For this review, use the dimensioned drawing (mm, ordinates from the lowest corner) and the shaded views. A direction names the side the tool comes from. Give positions to 0.01 mm unless a question says otherwise; leave off trailing zeros. Write each loop counter-clockwise with the first axis right and the second up, starting at its lowest first coordinate (ties: lowest second). Pieces come first, ordered by that corner, then holes. Notation, with made-up numbers: M -23.75,65.25 L 2.25,65.25 A22 ccw 2.25,103.25 Z; hole C 24.25,51.25 d6. An arc over 180 degrees is marked long. One line per item, written item: value. Start each with the question number.
Item 1: Consider section A-A, the plane x = 27.5. Write out the cut boundary in (y, z), and give its area (3 significant figures).
Item 2: Consider section B-B, the plane y = 15. Write out the cut boundary in (x, z), and give its area (3 significant figures).
Item 3: Tool access review of the marked faces 1 and 2: name each direction out of +Z, -Z, +X, -X, +Y, -Y from which nothing blocks a thin tool from reaching the whole face with its end or side.
Item 4: Mouldability with a two-part tool opening along X and no side actions: class the marked faces 3, 4 and 5 as released by +X, released by -X, zero draft, split by the parting line, or undercut.
Item 5: Clearance check with flat-ended pins moving along their axes: pin 1 Ø6 at (y, z) = (8.5, 13) entering from -X; pin 2 Ø11 at (x, y) = (15.5, 12.5) entering from -Z; pin 3 Ø6 at (x, y) = (5.5, 8.5) entering from +Z. State where each tip first meets the part, or that it passes through.
Item 6: Consider section D-D, the plane x = 15. Write out the cut boundary in (y, z), and give its area (3 significant figures).
Item 7: To check wall thickness, follow probe 1 along Y at (x, z) = (15, 7); probe 2 along Y at (x, z) = (23, 11); probe 3 along Z at (x, y) = (15.5, 13.5). State the ranges of each line that lie inside material, in increasing order.
Item 8: Consider section C-C, the plane z = 11. Write out the cut boundary in (x, y).
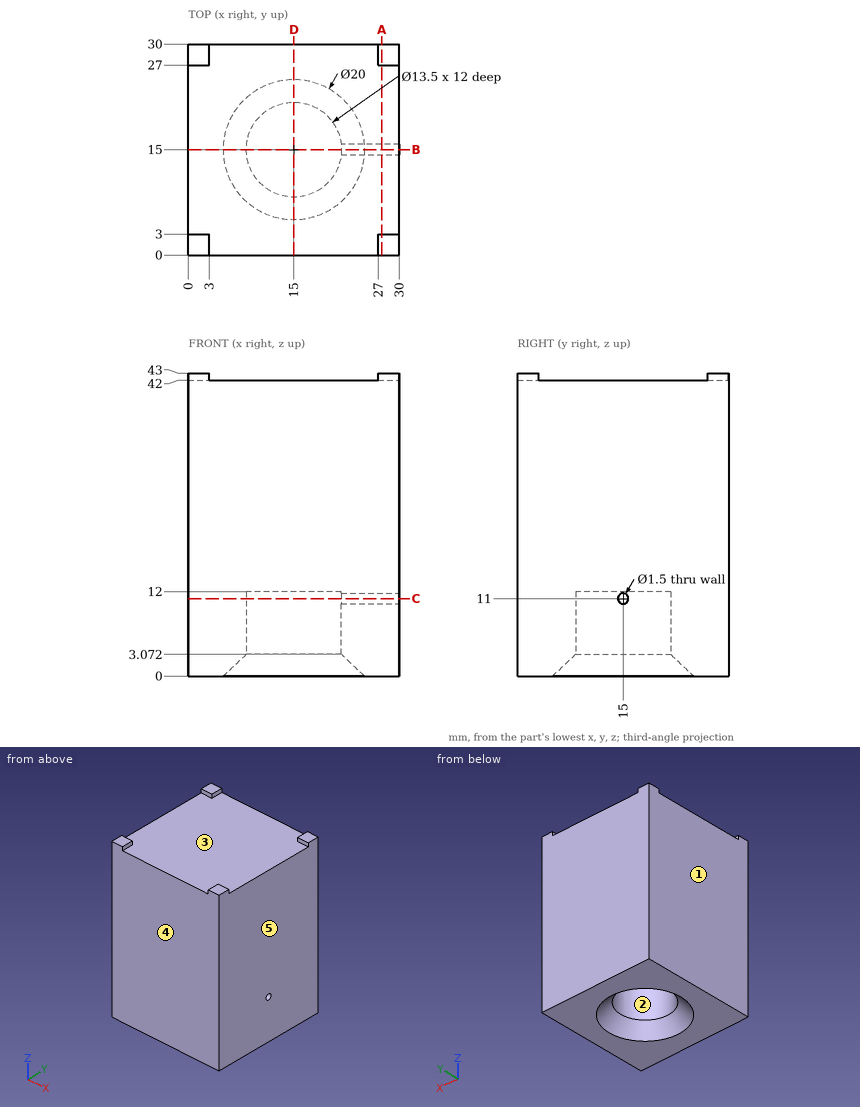
Model answer:
1. outline: M 0,0 L 30,0 L 30,43 L 27,43 L 27,42 L 3,42 L 3,43 L 0,43 Z; hole C 15,11 d1.5
1. area: 1,260 mm2
2. outline: M 0,0 L 5,0 L 8.25,3.07 L 8.25,12 L 21.75,12 L 21.75,11.75 L 30,11.75 L 30,42 L 0,42 Z; M 21.75,3.07 L 25,0 L 30,0 L 30,10.25 L 21.75,10.25 Z
2. area: 1,080 mm2
3. face 1: +Z, -Z, -X, +Y, -Y
3. face 2: -Z
4. face 3: undercut
4. face 4: zero draft
4. face 5: released by +X
5. pin 1: stops at x = 0
5. pin 2: stops at z = 1.84
5. pin 3: stops at z = 42
6. outline: M 0,0 L 5,0 L 8.25,3.07 L 8.25,12 L 21.75,12 L 21.75,3.07 L 25,0 L 30,0 L 30,42 L 0,42 Z
6. area: 1,090 mm2
7. probe 1: y = 0 to 8.25, 21.75 to 30
7. probe 2: y = 0 to 14.25, 15.75 to 30
7. probe 3: z = 12 to 42
8. outline: M 0,0 L 30,0 L 30,14.25 L 21.71,14.25 A6.75 cw long 21.71,15.75 L 30,15.75 L 30,30 L 0,30 Z
